Design review of the part shown in the three views and the two pictorial views. Dimensions are in mm from the part's minimum x, y and z. A direction names the side the tool comes from. Give positions to 0.01 mm unless a question says otherwise; leave off trailing zeros. Loops run counter-clockwise (first coordinate to the right, second up) from the corner with the lowest first, then second, coordinate; pieces in that order, holes last.
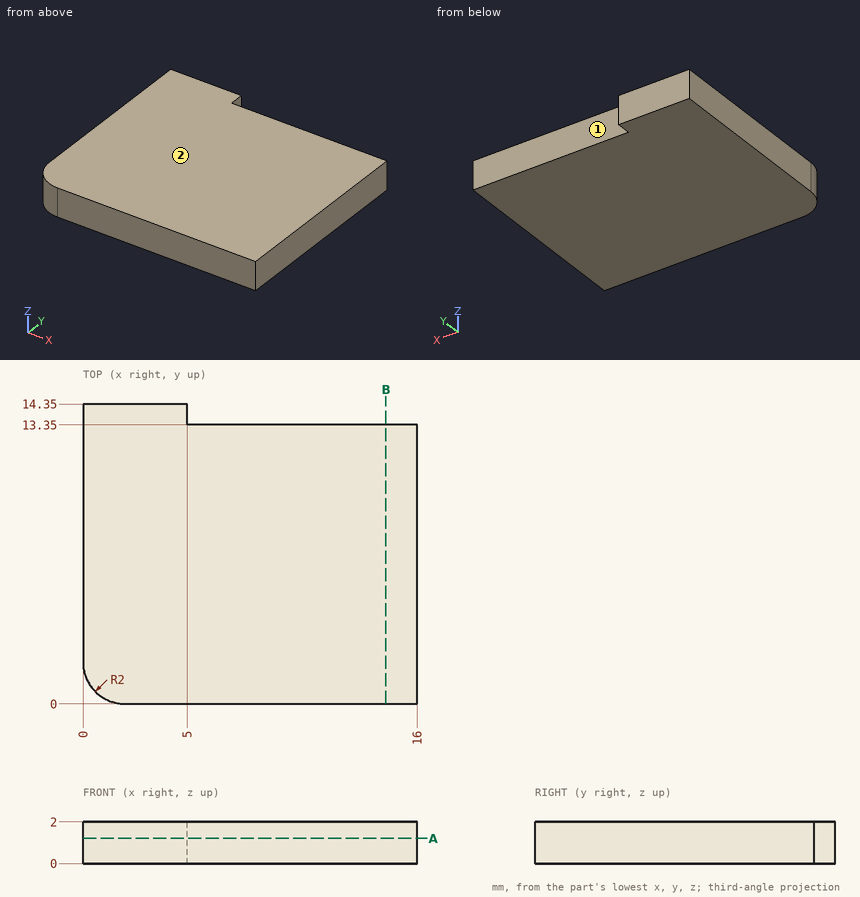
Q1. For probe 1 along X at (y, z) = (13.5, 1); probe 2 along Y at (x, z) = (14.75, 1.85); probe 3 along X at (y, z) = (0.75, 1.4), list the stretches that pass through material, from the lowest coordinate up.
Answers:
probe 1: x = 0 to 5
probe 2: y = 0 to 13.35
probe 3: x = 0.44 to 16
Q2. Consider section B-B on x = 14.5. Give the boundary of the cut face in (y, z), plus the area to 3 significant figures.
Answers:
outline: (0, 0) - (13.35, 0) - (13.35, 2) - (0, 2) - close
area: 26.7 mm2
Q3. Machinability: for the marked faces 1 and 2, which of the approach directions +Z, -Z, +X, -X, +Y, -Y give a long, thin tool a straight path to every point of the face, cutting with its end or side? Answer none if there is none.
Answers:
face 1: +Z, -Z, +X, +Y
face 2: +Z, +X, -X, +Y, -Y
Q4. Consider section A-A on z = 1.2. Give the boundary of the cut face in (x, y).
Answers:
outline: (0, 2) arc R2 ccw to (2, 0) - (16, 0) - (16, 13.35) - (5, 13.35) - (5, 14.35) - (0, 14.35) - close
